from build123d import *

# Parameters (mm, degrees)
SKETCH1_W           = 3.175
SKETCH1_H           = 20
BOSS_EXTRUDE1_DEPTH = 3.175
SKETCH10_W          = 3.09372
SKETCH10_H          = 19.91872
BOSS_EXTRUDE2_DEPTH = 3.175


with BuildPart() as part:
    # Sketch1 → Boss-Extrude1 (new body)
    with BuildSketch(Plane(origin=(0, 0, 0), x_dir=(1, 0, 0), z_dir=(0, 1, 0))):
        with BuildLine():
            Line((5.92993597, 290.47006403), (0, 296.4))
            Line((0, 296.4), (0, 0))
            Line((0, 0), (5.933366161, 5.951511012))
            ThreePointArc((5.933366161, 5.951511012), (5.242610834, 6.982741285), (5, 8.2))
            Line((5, 8.2), (5, 28.2))
            Line((5, 28.2), (8.175, 28.2))
            Line((8.175, 28.2), (8.175, 8.2))
            Line((8.175, 8.2), (13.175, 13.21529052))
            Line((13.175, 13.21529052), (13.175, 283.225))
            Line((13.175, 283.225), (8.175, 288.225))
            Line((8.175, 288.225), (8.175, 268.225))
            Line((8.175, 268.225), (5, 268.225))
            Line((5, 268.225), (5, 288.225))
            ThreePointArc((5, 288.225), (5.241682484, 289.440019898), (5.92993597, 290.47006403))
        make_face()
        with Locations((6.5875, 70.205)):
            Rectangle(SKETCH1_W, SKETCH1_H, mode=Mode.SUBTRACT)
        with Locations((6.5875, 122.21)):
            Rectangle(SKETCH1_W, SKETCH1_H, mode=Mode.SUBTRACT)
        with Locations((6.5875, 174.215)):
            Rectangle(SKETCH1_W, SKETCH1_H, mode=Mode.SUBTRACT)
        with Locations((6.5875, 226.22)):
            Rectangle(SKETCH1_W, SKETCH1_H, mode=Mode.SUBTRACT)
    extrude(amount=BOSS_EXTRUDE1_DEPTH)

    # Sketch10 → Boss-Extrude2 (add)
    with BuildSketch(Plane(origin=(0, 3.175, 0), x_dir=(1, 0, 0), z_dir=(0, 1, 0))):
        with BuildLine():
            Line((-0.04064, 296.498113639), (-0.04064, -0.098325868))
            Line((-0.04064, -0.098325868), (5.991025757, 5.95178535))
            ThreePointArc((5.991025757, 5.95178535), (5.287996872, 6.979579765), (5.04064, 8.2))
            Line((5.04064, 8.2), (5.04064, 28.15936))
            Line((5.04064, 28.15936), (8.13436, 28.15936))
            Line((8.13436, 28.15936), (8.13436, 8.101674132))
            Line((8.13436, 8.101674132), (13.21564, 13.198493215))
            Line((13.21564, 13.198493215), (13.21564, 283.241833639))
            Line((13.21564, 283.241833639), (8.13436, 288.323113639))
            Line((8.13436, 288.323113639), (8.13436, 268.26564))
            Line((8.13436, 268.26564), (5.04064, 268.26564))
            Line((5.04064, 268.26564), (5.04064, 288.225))
            ThreePointArc((5.04064, 288.225), (5.287066096, 289.443216062), (5.987595917, 290.469877722))
            Line((5.987595917, 290.469877722), (-0.04064, 296.498113639))
        make_face()
        with Locations((6.5875, 226.22)):
            Rectangle(SKETCH10_W, SKETCH10_H, mode=Mode.SUBTRACT)
        with Locations((6.5875, 174.215)):
            Rectangle(SKETCH10_W, SKETCH10_H, mode=Mode.SUBTRACT)
        with Locations((6.5875, 122.21)):
            Rectangle(SKETCH10_W, SKETCH10_H, mode=Mode.SUBTRACT)
        with Locations((6.5875, 70.205)):
            Rectangle(SKETCH10_W, SKETCH10_H, mode=Mode.SUBTRACT)
    extrude(amount=-BOSS_EXTRUDE2_DEPTH)


solid = part.part
For this review, take the finished solid that the model builds, in its own axes (mm). Coordinates: 2 decimals unless noted, no trailing zeros. Loops run counter-clockwise (first coordinate to the right, second up) from the corner with the lowest first, then second, coordinate; pieces in that order, holes last. Notation, with made-up numbers: (-25, 23.25) - (1, 23.25) arc R26 ccw to (1, 48.25) - close; hole circle Ø7 at (4, 6.5). An arc over 180 degrees is marked (long way). Use a Markdown table: item, result. Add a question column.
Item 1: We need section B-B (y = 1.5). Give the number of separate pieces and of enclosed holes in the cut face, and give its area (3 significant figures).
Item 2: For line 1 (Z direction, x = 7.25, y = 0.4); line 2 (X direction, y = 2.1, z = -274.5); line 3 (Z direction, x = 2, y = 0.25), list the stretches that pass through material, from the lowest coordinate up.
Item 3: We need section A-A (z = -124). Give the boundary of the cut face in (x, y) (3 decimals).
Item 4: Insertion check: pin 1 Ø1.5 at (x, y) = (6.5, 1.5) entering from +Z; pin 2 Ø1 at (x, y) = (2, 2) entering from +Z; pin 3 Ø0.9 at (x, y) = (6, 2) entering from +Z. Each pin has a flat end and moves straight along its axis. Give the tip position at first contact, or say it passes through.
Results list:
| question | item | result |
|---|---|---|
| 1 | separate pieces | 1 |
| 1 | enclosed holes | 4 |
| 1 | area | 3,380 mm^2 |
| 2 | line 1 | z = -268.27 to -236.18, -216.26 to -184.17, -164.26 to -132.17, -112.25 to -80.16, -60.25 to -28.16 |
| 2 | line 2 | x = -0.04 to 5.04, 8.13 to 13.22 |
| 2 | line 3 | z = -294.46 to -1.95 |
| 3 | outline | (-0.041, 0) - (5.041, 0) - (5.041, 3.175) - (-0.041, 3.175) - close; (8.134, 0) - (13.216, 0) - (13.216, 3.175) - (8.134, 3.175) - close |
| 4 | pin 1 | stops at z = -5.71 |
| 4 | pin 2 | stops at z = -1.45 |
| 4 | pin 3 | stops at z = -5.51 |
